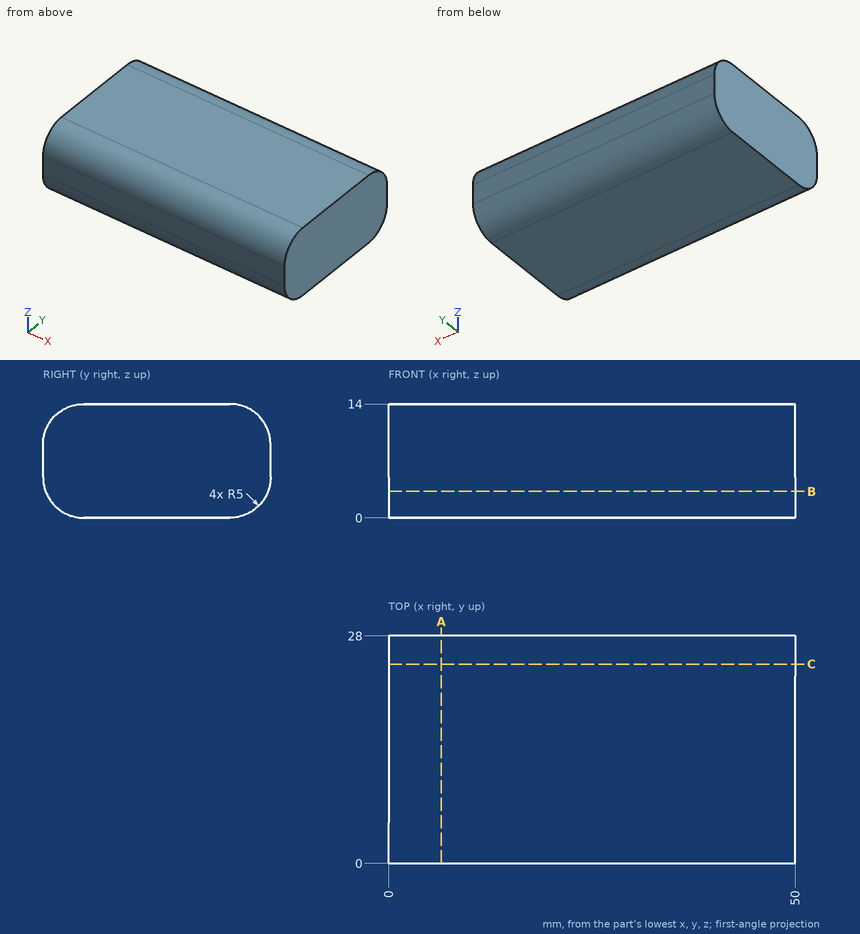
Study the drawing (mm; zero at the part's minimum x, y, z) and answer. Round coordinates to 2 decimals unless told otherwise and drop trailing zeros. Write each loop counter-clockwise with the first axis right and the second up, starting at its lowest first coordinate (ties: lowest second). Pieces come first, ordered by that corner, then holes.
1) Given pin 1 Ø4 at (x, y) = (25, 6) entering from -Z; pin 2 Ø1.5 at (x, z) = (36.5, 10.5) entering from -Y; pin 3 Ø1.5 at (x, z) = (10.5, 12.5) entering from -Y, each flat-ended and moving along its own axis, determine where each tip first touches the part or whether it passes through.
2) Straight lines are drawn through the part: line 1 (Z direction, x = 43, y = 23.25); line 2 (Y direction, x = 14, z = 9.25); line 3 (Y direction, x = 28, z = 12.75). For each, find the intervals that lie inside material, in ascending order.
3) A cutting plane is placed at C-C (y = 24.5). Give the vertices of the cut face in (x, z), plus the area to 3 significant figures.
4) A cutting plane is placed at A-A (x = 6.5). Give the vertices of the cut face in (y, z).
5) A cutting plane is placed at B-B (z = 3.25). Give the vertices of the cut face in (x, y).
Completed:
1. pin 1: stops at z = 0
1. pin 2: stops at y = 0.06
1. pin 3: stops at y = 0.82
2. line 1: z = 0.01 to 13.99
2. line 2: y = 0.01 to 27.99
2. line 3: y = 1.69 to 26.31
3. outline: (0, 0.23) - (50, 0.23) - (50, 13.77) - (0, 13.77) - close
3. area: 677 mm2
4. outline: (0, 5) arc R5 ccw to (5, 0) - (23, 0) arc R5 ccw to (28, 5) - (28, 9) arc R5 ccw to (23, 14) - (5, 14) arc R5 ccw to (0, 9) - close
5. outline: (0, 0.32) - (50, 0.32) - (50, 27.68) - (0, 27.68) - close
